Geometry check sheet. Reference: drawing and pictorial views, mm from the part's lowest x, y, z. A direction names the side the tool comes from. Coordinates: 2 decimals unless noted, no trailing zeros. Loops run counter-clockwise (first coordinate to the right, second up) from the corner with the lowest first, then second, coordinate; pieces in that order, holes last. Notation, with made-up numbers: (-23.5, -36.5) -> (-12.5, -36.5) arc R30 ccw to (-12.5, -9.5) -> close; hole circle Ø6 at (82.25, 65). An arc over 180 degrees is marked (long way). Use one line per item in the form item = value.
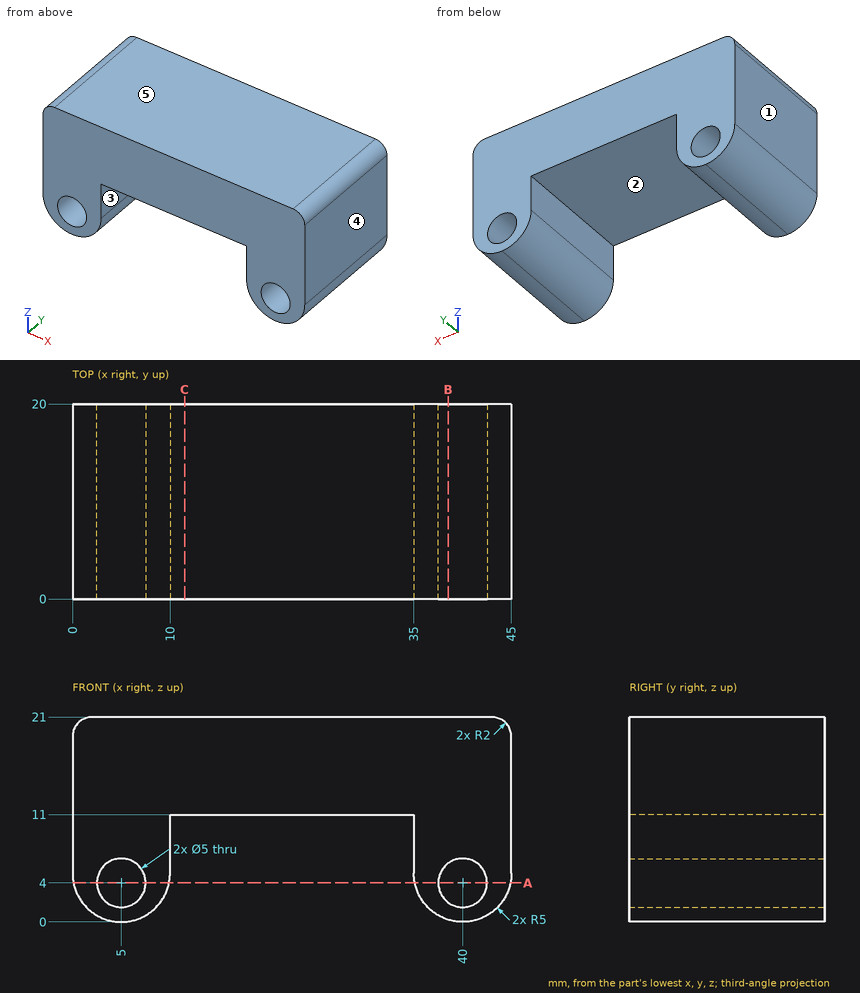
(1) Section check A-A, the plane z = 4. Record the boundary of the cut face in (x, y).
Established:
outline = (0.1, 0) -> (2.5, 0) -> (2.5, 20) -> (0.1, 20) -> close; (7.5, 0) -> (9.9, 0) -> (9.9, 20) -> (7.5, 20) -> close; (35.1, 0) -> (37.5, 0) -> (37.5, 20) -> (35.1, 20) -> close; (42.5, 0) -> (44.9, 0) -> (44.9, 20) -> (42.5, 20) -> close
(2) Scan lines: line 1 along X through (y, z) = (1.25, 6.75); line 2 along Z through (x, y) = (5, 11.75); line 3 along Z through (x, y) = (31, 18.5). Record each from-to range of solid material in increasing order.
Established:
line_1 = 0 to 10, 35 to 45
line_2 = 0 to 1.5, 6.5 to 21
line_3 = 11 to 21
(3) Section check C-C, the plane x = 11.5. Record the boundary of the cut face in (y, z).
Established:
outline = (0, 11) -> (20, 11) -> (20, 21) -> (0, 21) -> close
(4) Go/stop test with a flat-tipped pin: P1, Ø6, axis at x = 31.5, y = 13, coming from the -Z side. Record where the tip stops, or that it passes through.
Established:
P1 = 11
(5) Mould release check, pull along X, two halves, no side actions. Record for the marked faces 3, 4 and 5: +X half, -X half, draft (parallel to the pull), parting line (faces both ways), or undercut.
Established:
face_3 = undercut
face_4 = +X half
face_5 = draft
(6) Section check B-B, the plane x = 38.5. Record the boundary of the cut face in (y, z), plus the area to 3 significant figures.
Established:
outline = (0, 0.23) -> (20, 0.23) -> (20, 2) -> (0, 2) -> close; (0, 6) -> (20, 6) -> (20, 21) -> (0, 21) -> close
area = 335 mm²
(7) Tool access check on the marked faces 1 and 2. Record the directions out of +Z, -Z, +X, -X, +Y, -Y that give a thin tool (end or side, any length) a straight path to the whole face; none if there is none.
Established:
face_1 = +Z, -Z, -X, +Y, -Y
face_2 = -Z, +Y, -Y
